Can you work these out from the model? Positions are in its coordinate system, mm. Coordinates: 2 decimals unless noted, no trailing zeros. Order: outer loops, then holes, each group sorted by start corner. A loop starts at its lowest first (then second) coordinate and runs counter-clockwise, first axis right, second up. Notation, with made-up numbers: M 31.5,31.25 L 44.5,31.25 A15 cw 44.5,40.25 Z; hole C 15.5,50 d1. An arc over 180 degrees is marked long. Answer as CSV lines item,"result". Start each with the question number.
1. Will these pins go through, and if not, where does the flat tip stop? pin 1 (6 mm diameter, centred on x = 5.5, z = -82.5, fed in from +Y); pin 2 (5 mm diameter, centred on x = 6, z = -22, fed in from +Y); pin 3 (11 mm diameter, centred on y = -18, z = -247, fed in from -X); pin 4 (4 mm diameter, centred on x = 1.5, y = 1.5, fed in from -Z).
2. If we section it at D-D (z = -116.5): List the corners of the cut face in (x, y) for me, plus the area to 3 significant figures.
3. If we section it at A-A (z = -247): List the corners of the cut face in (x, y) for me, plus the area to 3 significant figures.
4. If we section it at B-B (y = -18): List the corners of the cut face in (x, z) for me, plus the area to 3 significant figures.
5. If we section it at C-C (x = 5.5): List the corners of the cut face in (y, z) for me.
6. I need wall thicknesses on line 1 along Y through (x, z) = (7.5, -247); line 2 along Z through (x, y) = (8.5, -21.5); line 3 along Z through (x, y) = (1.5, -24). Which ranges of each line are inside material? Lowest first, please. Write a range as from..to.
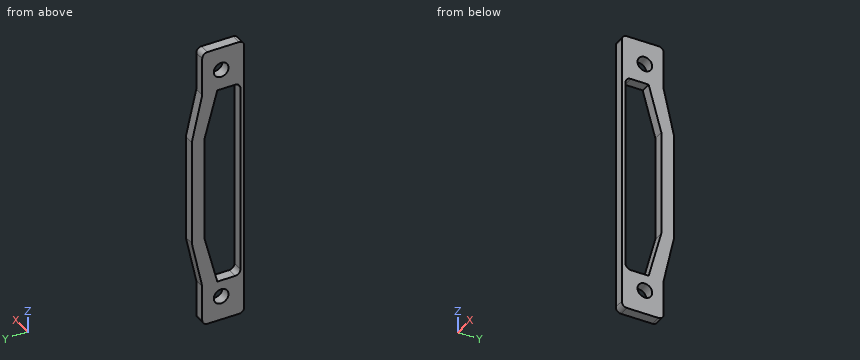
Autodesk Inventor part; units mm, degrees
ref_plane "YZ Plane" through (0, 0, 0) normal (1, 0, 0) x (0, 1, 0)
ref_plane "XZ Plane" through (0, 0, 0) normal (0, 1, 0) x (-1, 0, 0)
ref_plane "XY Plane" through (0, 0, 0) normal (0, 0, 1) x (1, 0, 0)
sketch "Sketch2" plane through (0, 0, 0) normal (1, 0, 0) x (0, 1, 0)
  line L0 (0, 0) -> (-40, 0)
  line L1 (-40, 0) -> (-40, -270)
  line L2 (-40, -270) -> (0, -270)
  line L3 (0, -270) -> (0, 0)
  dimension "d0" = 40
  dimension "d1" = 270
extrude "Extrusion1" add sketch "Sketch2" along normal blind 10
sketch "Sketch3" plane through (10, 0, 0) normal (1, 0, 0) x (0, 0, -1)
  circle A0 centre (22, -18) radius 7
  line L0 (270, 0) -> (0, 0)
  dimension "d4" = 14
  dimension "d10" = 18
extrude "Extrusion2" cut sketch "Sketch3" against normal through all
sketch "Sketch4" plane through (10, 0, 0) normal (1, 0, 0) x (0, 0, -1)
  circle A0 centre (247, -18) radius 7
  line L0 (270, 0) -> (0, 0)
  dimension "d7" = 14
  dimension "d11" = 18
extrude "Extrusion3" cut sketch "Sketch4" against normal through all
sketch "Sketch5" plane through (10, 0, 0) normal (1, 0, 0) x (0, 0, -1)
  line L0 (41.1855, -36.3701) -> (231.1855, -36.3701)
  line L1 (231.1855, -36.3701) -> (231.1855, -14.3701)
  line L2 (231.1855, -14.3701) -> (41.1855, -14.3701)
  line L3 (41.1855, -14.3701) -> (41.1855, -36.3701)
  point P0 (0, 0)
  dimension "d14" = 22
  dimension "d15" = 190
extrude "Extrusion4" cut sketch "Sketch5" against normal through all
sketch "Sketch15" plane through (10, 0, 0) normal (1, 0, 0) x (0, 0, -1)
  line L0 (135, 10) -> (85, 10)
  line L1 (85, 10) -> (185, 10)
  line L2 (185, 10) -> (231.1855, 0)
  line L3 (270, 0) -> (0, 0)
  line L4 (85, 10) -> (41.1855, 0)
  line L5 (41.1855, -36.3701) -> (41.1855, -14.3701)
  line L6 (41.1855, -14.3701) -> (85, 0)
  line L7 (185, 0) -> (231.1855, -12.1069)
  point P0 (41.1855, -30)
  dimension "d37" = 50
  dimension "d38" = 100
extrude "Extrusion10" add sketch "Sketch15" against normal blind 10
sketch "Sketch16" plane through (10, 0, 0) normal (1, 0, 0) x (0, 0, -1)
  line L0 (41.1855, -14.3701) -> (231.1855, -14.3701)
  line L1 (41.1855, -14.3701) -> (85, -2.2632)
  line L2 (85, -2.2632) -> (185, -2.2632)
  line L3 (85, 10) -> (185, 10)
  line L4 (185, -2.2632) -> (231.1855, -14.3701)
  point P0 (0, 0)
extrude "Extrusion11" cut sketch "Sketch16" against normal through all
fillet "Fillet1" radius 5 6 edges at (5, -40, 0) (5, 0, 0) (5, -40, -270) (5, 0, -270) (5, -36.3701, -231.1855) (5, -36.3701, -41.1855)
properties part number "estructura union gusano"
Solved:
1,pin 1,"y = 10"
1,pin 2,"y = 0"
1,pin 3,"through"
1,pin 4,"z = -267.18"
2,outline,"M 0,-40 L 10,-40 L 10,-36.37 L 0,-36.37 Z; M 0,-2.26 L 10,-2.26 L 10,10 L 0,10 Z"
2,area,"159 mm²"
3,outline,"M 0,-40 L 10,-40 L 10,-25 L 0,-25 Z; M 0,-11 L 10,-11 L 10,0 L 0,0 Z"
3,area,"260 mm²"
4,outline,"M 0,-270 L 10,-270 L 10,-254 L 0,-254 Z; M 0,-240 L 10,-240 L 10,-231.19 L 0,-231.19 Z; M 0,-41.19 L 10,-41.19 L 10,-29 L 0,-29 Z; M 0,-15 L 10,-15 L 10,0 L 0,0 Z"
4,area,"520 mm²"
5,outline,"M -40,-265 A5 ccw -35,-270 L -5,-270 A5 ccw 0,-265 L 0,-231.19 L 10,-185 L 10,-85 L 0,-41.19 L 0,-5 A5 ccw -5,0 L -35,0 A5 ccw -40,-5 Z; hole M -36.37,-226.19 A5 ccw -31.37,-231.19 L -14.37,-231.19 L -2.26,-185 L -2.26,-85 L -14.37,-41.19 L -31.37,-41.19 A5 ccw -36.37,-46.19 Z; hole C -18,-247 d14; hole C -18,-22 d14"
6,line 1,"-40..-25, -11..0"
6,line 2,"-270..-253.06, -240.94..-231.19, -41.19..-28.06, -15.94..0"
6,line 3,"-270..-250.61, -243.39..-231.19, -41.19..-25.61, -18.39..0"
